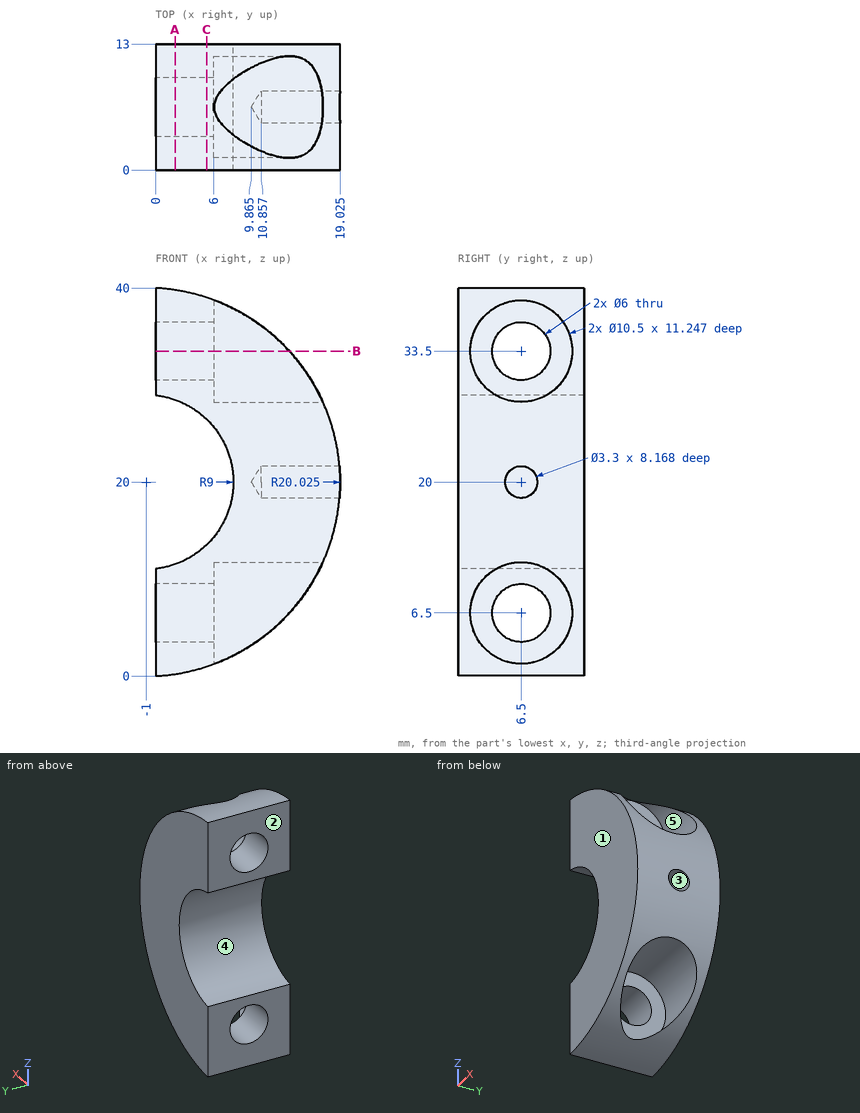
Source: three-view drawing plus pictorial views. Frame: mm from the lowest corner of the part. A direction names the side the tool comes from. Coordinates: 2 decimals unless noted, no trailing zeros. Loops run counter-clockwise (first coordinate to the right, second up) from the corner with the lowest first, then second, coordinate; pieces in that order, holes last. Notation, with made-up numbers: (20, 40.5) -> (25, 40.5) arc R26 cw to (25, 65.5) -> close; hole circle Ø8 at (81, -28.5). An arc over 180 degrees is marked (long way). One line per item, written item: value.
(1) Draft query along Y for the marked faces 1, 2 and 3. Return one class per face: pulls with the +Y half, pulls with the -Y half, needs draft (parallel to the pull), parting line crosses it, or undercut.
Answer below:
face 1: pulls with the -Y half
face 2: needs draft
face 3: undercut
(2) Ray query, line 1 along Z through (x, y) = (3, 7.75); line 2 along Z through (x, y) = (1.75, 6) (1 decimal); line 3 along Z through (x, y) = (9.75, 2) (1 decimal). Return the intervals inside material, ascending.
Answer below:
line 1: z = 0.38 to 3.77, 9.23 to 11.94, 28.06 to 30.77, 36.23 to 39.62
line 2: z = 0.2 to 3.5, 9.5 to 11.4, 28.6 to 30.5, 36.5 to 39.8
line 3: z = 3.1 to 3.8, 9.2 to 30.8, 36.2 to 36.9
(3) Cut plane C-C (x = 5.25). Output: boundary loops of the cut face in (y, z) (1 decimal), then the cut area to 3 significant figures.
Answer below:
outline: (0, 1) -> (13, 1) -> (13, 13.5) -> (0, 13.5) -> close; (0, 26.5) -> (13, 26.5) -> (13, 39) -> (0, 39) -> close; hole circle Ø6 at (6.5, 6.5); hole circle Ø6 at (6.5, 33.5)
area: 270 mm2
(4) Cut plane B-B (z = 33.5). Output: boundary loops of the cut face in (x, y).
Answer below:
outline: (0, 0) -> (13.79, 0) -> (13.79, 1.25) -> (6, 1.25) -> (6, 3.5) -> (0, 3.5) -> close; (0, 9.5) -> (6, 9.5) -> (6, 11.75) -> (13.79, 11.75) -> (13.79, 13) -> (0, 13) -> close
(5) Pin query (flat end, axial travel): pin 1 Ø3.5 at (y, z) = (6.5, 33.5) entering from +X; pin 2 Ø1.5 at (x, y) = (7, 5.5) entering from -Z; pin 3 Ø3 at (y, z) = (4.5, 32.5) entering from +X; pin 4 Ø1.5 at (x, y) = (12, 3) entering from +Z. Return the tip coordinate at first contact, or that it passes through.
Answer below:
pin 1: passes through
pin 2: stops at z = 1.33
pin 3: stops at x = 6
pin 4: stops at z = 30.42
(6) Set-up query: the marked faces 4 and 5. Return all of +Z, -Z, +X, -X, +Y, -Y with unobstructed straight access to the full face (end or side cutting, diameter ignored); none if empty.
Answer below:
face 4: -X, +Y, -Y
face 5: +X
(7) Cut plane A-A (x = 2). Output: boundary loops of the cut face in (y, z) (1 decimal).
Answer below:
outline: (0, 0.2) -> (13, 0.2) -> (13, 11.5) -> (0, 11.5) -> close; (0, 28.5) -> (13, 28.5) -> (13, 39.8) -> (0, 39.8) -> close; hole circle Ø6 at (6.5, 6.5); hole circle Ø6 at (6.5, 33.5)
